from build123d import *

# Parameters (mm, degrees)
SKETCH_W     = 62
SKETCH_H     = 30
SKETCH_R     = 2.25
PAD_DEPTH    = 7
SKETCH001_R  = 3.8
POCKET_DEPTH = 3
FILLET_R     = 11
CHAMFER_SIZE = 2


with BuildPart() as part:
    # Sketch → Pad (new body)
    with BuildSketch(Plane.XY):
        Rectangle(SKETCH_W, SKETCH_H)
        with Locations((-25, 0)):
            Circle(SKETCH_R, mode=Mode.SUBTRACT)
        with Locations((25, 0)):
            Circle(SKETCH_R, mode=Mode.SUBTRACT)
        with Locations((0, 10)):
            Circle(SKETCH_R, mode=Mode.SUBTRACT)
        with Locations((0, -10)):
            Circle(SKETCH_R, mode=Mode.SUBTRACT)
    extrude(amount=PAD_DEPTH)

    # Sketch001 → Pocket (cut)
    with BuildSketch(Plane.XY.offset(7)):
        with Locations((0, 10)):
            Circle(SKETCH001_R)
        with Locations((0, -10)):
            Circle(SKETCH001_R)
    extrude(amount=-POCKET_DEPTH, mode=Mode.SUBTRACT)

    # Fillet
    fillet_edges = [part.edges().sort_by_distance(p)[0] for p in [
        (31, 15, 3.5),
        (-31, 15, 3.5),
        (-31, -15, 3.5),
        (31, -15, 3.5),
    ]]
    fillet(fillet_edges, radius=FILLET_R)

    # Chamfer
    chamfer_edges = [part.edges().sort_by_distance(p)[0] for p in [
        (0, 15, 0),
    ]]
    chamfer(chamfer_edges, length=CHAMFER_SIZE)


solid = part.part
Input: part model. Units: mm. Frame: model coordinates. A direction names the side the tool comes from. Give positions to 0.01 mm unless a question says otherwise; leave off trailing zeros. Write each loop counter-clockwise with the first axis right and the second up, starting at its lowest first coordinate (ties: lowest second). Pieces come first, ordered by that corner, then holes.
Q1. Section C-C, the plane z = 5.25. Output: boundary loops of the cut face in (x, y), plus the area to 3 significant figures.
Q2. Section B-B, the plane y = 0. Output: boundary loops of the cut face in (x, z).
Q3. First-contact query: P1, Ø10, axis at x = 0, y = -10, coming from the -Z side; P2, Ø5, axis at x = 0, y = 10, coming from the +Z side; P3, Ø2.5, axis at x = 0, y = 10.5, coming from the +Z side; P4, Ø4, axis at y = -12, z = 4, coming from the +X side. Flat tips, straight axial feed; report the tip coordinate or a pass-through.
Q4. Section D-D, the plane x = -14. Output: boundary loops of the cut face in (y, z), plus the area to 3 significant figures.
Q5. Set-up query: faces 4 (the face through (31, 0, 4)), 5 (the face through (2, -12, 4)). Return all of +Z, -Z, +X, -X, +Y, -Y with unobstructed straight access to the full face (end or side cutting, diameter ignored); none if empty.
Q6. Material intervals for probe 1 along Y at (x, z) = (0, 2.9); probe 2 along Y at (x, z) = (0, 6); probe 3 along Y at (x, z) = (-25, 3), sorted ascending.
Q7. Pull-direction query (X, two-part tool) for faces 1 (the face through (27.692, -11.863, 4.535)), 2 (the face through (2, 8, 4)), 3 (the face through (-27.863, 11.692, 4.535)); classes: pulls with the +X half, pulls with the -X half, needs draft (parallel to the pull), parting line crosses it, or undercut.
Q8. Section A-A, the plane x = 0. Output: boundary loops of the cut face in (y, z).
Filled in:
1. outline: (-31, -4) arc R11 ccw to (-20, -15) - (20, -15) arc R11 ccw to (31, -4) - (31, 4) arc R11 ccw to (20, 15) - (-20, 15) arc R11 ccw to (-31, 4) - close; hole circle Ø4.5 at (-25, 0); hole circle Ø7.6 at (0, -10); hole circle Ø7.6 at (0, 10); hole circle Ø4.5 at (25, 0)
1. area: 1,630 mm2
2. outline: (-31, 2) - (-29, 0) - (-27.25, 0) - (-27.25, 7) - (-31, 7) - close; (-22.75, 0) - (22.75, 0) - (22.75, 7) - (-22.75, 7) - close; (27.25, 0) - (29, 0) - (31, 2) - (31, 7) - (27.25, 7) - close
3. P1: stops at z = 0
3. P2: stops at z = 4
3. P3: passes through
3. P4: stops at x = 29.22
4. outline: (-15, 2) - (-13, 0) - (13, 0) - (15, 2) - (15, 7) - (-15, 7) - close
4. area: 206 mm2
5. face 4: +Z, -Z, +X, +Y, -Y
5. face 5: +Z
6. probe 1: y = -15 to -12.25, -7.75 to 7.75, 12.25 to 15
6. probe 2: y = -15 to -13.8, -6.2 to 6.2, 13.8 to 15
6. probe 3: y = -13.8 to -2.25, 2.25 to 13.8
7. face 1: pulls with the +X half
7. face 2: undercut
7. face 3: pulls with the -X half
8. outline: (-15, 2) - (-13, 0) - (-12.25, 0) - (-12.25, 4) - (-13.8, 4) - (-13.8, 7) - (-15, 7) - close; (-7.75, 0) - (7.75, 0) - (7.75, 4) - (6.2, 4) - (6.2, 7) - (-6.2, 7) - (-6.2, 4) - (-7.75, 4) - close; (12.25, 0) - (13, 0) - (15, 2) - (15, 7) - (13.8, 7) - (13.8, 4) - (12.25, 4) - close
